Autodesk Inventor part; units mm, degrees
ref_plane "screwMaxDist" through (2.525, 0, 1.825) normal (0, 0, 1) x (1, 0, 0)
ref_plane "YZ Plane" through (0, 0, 0) normal (1, 0, 0) x (0, 1, 0)
ref_plane "XZ Plane" through (0, 0, 0) normal (0, 1, 0) x (-1, 0, 0)
sketch "Sketch1" plane through (0, 0, 0) normal (0, 1, 0) x (-1, 0, 0)
  circle A0 centre (-2.525, 2.525) radius 1.2
  circle A1 centre (-2.525, 2.525) radius 2.525
  line L0 (0, 0) -> (-7.3028, 0) construction
  line L1 (0, 0) -> (0, 4.3038) construction
  dimension "d0" = 2.4
  dimension "d1" = 5.05
extrude "Extrusion1" add sketch "Sketch1" along normal blind 9
ref_plane "Work Plane1" through (2.525, 0, 1.325) normal (0, 0, 1) x (1, 0, 0)
ref_plane "screwMaxDist" through (2.525, 0, 1.825) normal (0, 0, 1) x (1, 0, 0)
sketch "Sketch2" plane through (0, 0, 0) normal (0, 0, 1) x (1, 0, 0)
  line L0 (5.05, 9) -> (0, 9)
  circle A0 centre (2.525, 4.8) radius 2.2
  line L1 (5.05, 9) -> (0, 9)
  line L2 (5.05, 0) -> (0, 0)
  line L3 (0, 0) -> (0, 9)
  line L4 (0, 7) -> (5.05, 7)
  line L5 (5.05, 0) -> (5.05, 9)
  dimension "d5" = 4.4
  dimension "d15" = 2
  dimension "d16" = 2.525
  dimension "d17" = 2.525
extrude "Extrusion2" cut sketch "Sketch2" along normal up to surface (1.825 mm away) contours A0
fillet "Fillet1" radius 0.2 4 edges at (3.725, 9, 2.525) (3.725, 0, 2.525) (5.05, 9, 2.525) (5.05, 0, 2.525)
equation "\"d16\" = d17"
properties part number "motor_shaft_adapter" material "ABS Plastic"
Can you work these out from the model? Positions are in its coordinate system, mm. A direction names the side the tool comes from. Round coordinates to 2 decimals unless told otherwise and drop trailing zeros. Order: outer loops, then holes, each group sorted by start corner. A loop starts at its lowest first (then second) coordinate and runs counter-clockwise, first axis right, second up. Notation, with made-up numbers: (46, 19.5) -> (77, 19.5) arc R6 ccw to (77, 27.5) -> close; hole circle Ø6 at (69, 51). An arc over 180 degrees is marked (long way). Write each question's results on one line, items separated by ' | '. Start each with the question number.
Item 1: If we section it at B-B, the plane x = 3.3: State how many separate pieces and enclosed holes the cut face has, then the cut area to 3 significant figures.
Item 2: Which directions (+Z, -Z, +X, -X, +Y, -Y) give clear straight access to the entire face, cutting with the end or side of a thin tool? Please do faces 5 (the cylindrical face through (2.785, 4.44, 3.696)), 6 (the flat face through (4, 5, 1.825)).
Item 3: Thinking about a two-plate mould opening in X: for faces 1 (the cylindrical face through (3.54, 6.75, 1.1)), 2 (the flat face through (1, 9, 3)), 3 (the cylindrical face through (3.07, 4.44, 4.99)), 4 (the flat face through (1, 5, 1.825)), which applies, +X half, -X half, draft (parallel to the pull), parting line (faces both ways), or undercut?
Item 4: Please list where these lines run through material, in increasing order: L1, parallel to X at y = 3.25, z = 2.45; L2, parallel to X at y = 1.25, z = 1.7.
Item 5: If we section it at A-A, the plane y = 5.25: Write out the boundary of the cut face in (x, z) (3 decimals), then the cut area to 3 significant figures.
Item 6: Will this pin go through, and if not, where does the flat tip stop? pin 1 (1.3 mm diameter, centred on x = 4.5, y = 4.5, fed in from -Z).
Item 7: If we section it at C-C, the plane y = 2: Write out the boundary of the cut face in (x, z) (3 decimals).
Results:
1) separate pieces: 3 | enclosed holes: 0 | area: 20.6 mm2
2) face 5: +Y, -Y | face 6: -Z
3) face 1: undercut | face 2: draft | face 3: parting line | face 4: undercut
4) L1: x = 0 to 1.33, 3.72 to 5.05 | L2: x = 0.14 to 1.65, 3.4 to 4.91
5) outline: (0.372, 1.207) -> (0.372, 1.825) -> (1.55, 1.825) arc R1.2 cw (long way) to (3.5, 1.825) -> (4.678, 1.825) -> (4.678, 1.207) arc R2.525 ccw (long way) to start | area: 9.85 mm2
6) pin 1: stops at z = 0.96
7) outline: circle Ø5.05 at (2.525, 2.525); hole circle Ø2.4 at (2.525, 2.525)
